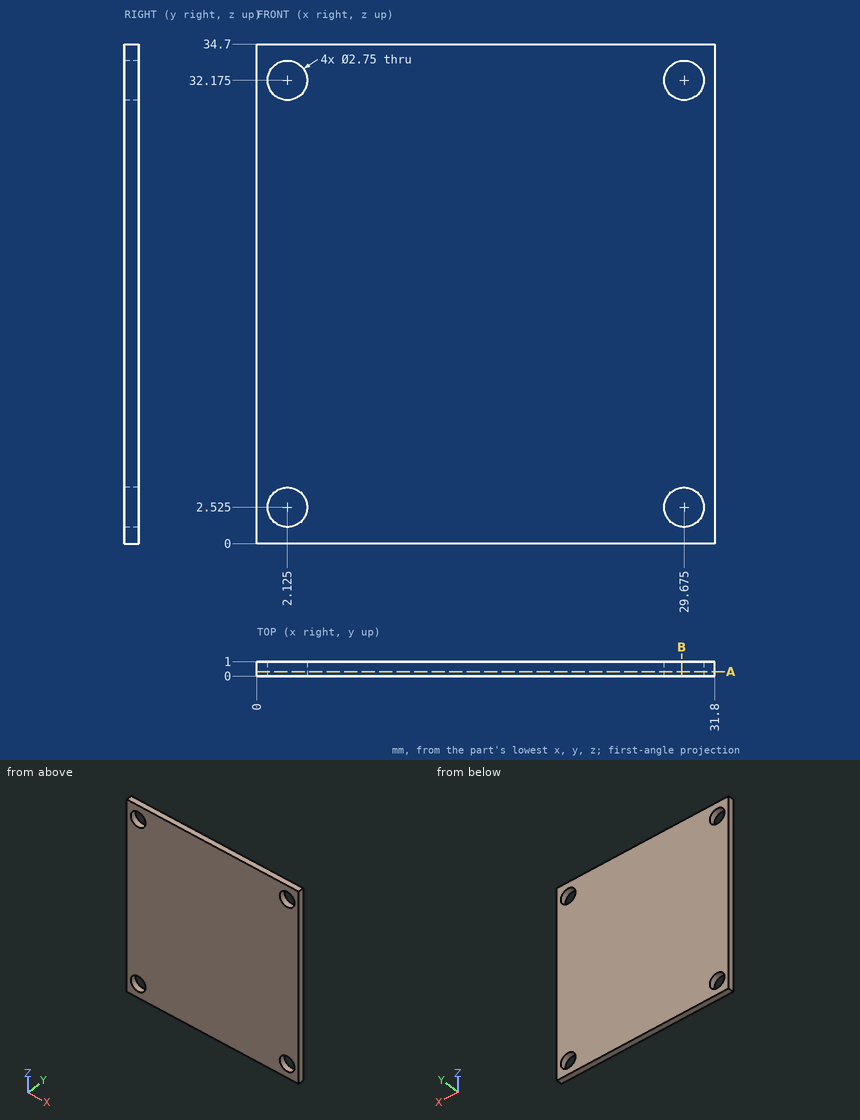
Design review of the part shown in the three views and the two pictorial views. Dimensions are in mm from the part's minimum x, y and z. Give positions to 0.01 mm unless a question says otherwise; leave off trailing zeros. Write each loop counter-clockwise with the first axis right and the second up, starting at its lowest first coordinate (ties: lowest second). Pieces come first, ordered by that corner, then holes. Notation, with made-up numbers: M 35,73 L 77,73 A20 cw 77,88 Z; hole C 55.25,-4 d10. An arc over 180 degrees is marked long. Answer as CSV lines item,"result".
1. Consider section A-A, the plane y = 0.3. Write out the cut boundary in (x, z) (3 decimals).
Findings:
outline,"M 0,0 L 31.8,0 L 31.8,34.7 L 0,34.7 Z; hole C 2.125,2.525 d2.75; hole C 2.125,32.175 d2.75; hole C 29.675,2.525 d2.75; hole C 29.675,32.175 d2.75"
2. Consider section B-B, the plane x = 29.5. Write out the cut boundary in (y, z), then the cut area to 3 significant figures.
Findings:
outline,"M 0,0 L 1,0 L 1,1.16 L 0,1.16 Z; M 0,3.89 L 1,3.89 L 1,30.81 L 0,30.81 Z; M 0,33.54 L 1,33.54 L 1,34.7 L 0,34.7 Z"
area,"29.2 mm2"
3. For pin 1 (4.5 mm diameter, centred on x = 29.675, z = 32.175, fed in from -Y); pin 2 (2.5 mm diameter, centred on x = 2.125, z = 32.175, fed in from +Y), all flat-tipped, find the tip position at first contact; note any pin that passes through.
Findings:
pin 1,"stops at y = 0"
pin 2,"passes through"
4. Wall thickness on line 1 (Z direction, x = 30.5, y = 0.3) (3 decimals); line 2 (Z direction, x = 28.5, y = 0.6); line 3 (X direction, y = 0.9, z = 33) (3 decimals): over which ranges is each line inside the solid? List them lowest first.
Findings:
line 1,"z = 0 to 1.425, 3.625 to 31.075, 33.275 to 34.7"
line 2,"z = 0 to 1.81, 3.24 to 31.46, 32.89 to 34.7"
line 3,"x = 0 to 1.025, 3.225 to 28.575, 30.775 to 31.8"
